Autodesk Inventor part; units mm, degrees
ref_plane "YZ Plane" through (0, 0, 0) normal (1, 0, 0) x (0, 1, 0)
ref_plane "XZ Plane" through (0, 0, 0) normal (0, 1, 0) x (-1, 0, 0)
ref_plane "XY Plane" through (0, 0, 0) normal (0, 0, 1) x (1, 0, 0)
sketch "Sketch1" plane through (0, 0, 0) normal (0, 1, 0) x (-1, 0, 0)
  point P0 (0, 0)
sketch "Sketch2" plane through (0, 0, 0) normal (0, 1, 0) x (-1, 0, 0)
  line L0 (0, 0) -> (104.775, 0)
  line L1 (104.775, 0) -> (104.775, -249.2375)
  line L2 (104.775, -249.2375) -> (0, -249.2375)
  line L3 (0, -249.2375) -> (0, 0)
  dimension "d0" = 104.775
  dimension "d1" = 249.2375
extrude "Extrusion1" add sketch "Sketch2" along normal blind 1.5875
sketch "Sketch3" plane through (0, 1.5875, 0) normal (0, 1, 0) x (1, 0, 0)
  line L0 (-104.775, 0) -> (0, 0)
  line L1 (-104.775, 0) -> (-103.1875, 0)
  line L2 (-103.1875, 0) -> (-103.1875, 304.8)
  line L3 (-104.775, 304.8) -> (-104.775, 0)
  line L4 (-104.775, 249.2375) -> (-104.775, 0)
  line L5 (-104.775, 0) -> (79.375, 0)
  line L6 (79.375, 0) -> (79.375, 1.5875)
  line L7 (79.375, 1.5875) -> (-104.775, 1.5875)
  line L8 (-104.775, 1.5875) -> (-104.775, 0)
  line L9 (0, 249.2375) -> (-104.775, 249.2375)
  line L10 (-104.775, 249.2375) -> (79.375, 249.2375)
  line L11 (79.375, 249.2375) -> (79.375, 247.65)
  line L12 (79.375, 247.65) -> (-104.775, 247.65)
  line L13 (-104.775, 247.65) -> (-104.775, 249.2375)
  line L14 (-104.775, 304.8) -> (-103.1875, 304.8)
  line L15 (-103.1875, 304.8) -> (-103.1875, 0)
  line L16 (-103.1875, 0) -> (-104.775, 0)
  line L17 (-104.775, 0) -> (-104.775, 304.8)
  dimension "d6" = 184.15
  dimension "d7" = 1.5875
  dimension "d8" = 184.15
  dimension "d9" = 1.5875
  dimension "d10" = 1.5875
  dimension "d11" = 304.8
extrude "Extrusion2" add sketch "Sketch3" along normal blind 76.2
sketch "Sketch4" plane through (-103.1875, 1.5875, -1.5875) normal (1, 0, 0) x (0, 0, -1)
  line L0 (-1.5875, -1.5875) -> (-1.5875, 0) construction
  line L1 (-1.5875, -1.5875) -> (30.1625, -1.5875) construction
  line L2 (247.65, -1.5875) -> (-1.5875, -1.5875) construction
  line L3 (30.1625, -1.5875) -> (30.1625, 0) construction
  line L4 (0, 0) -> (246.0625, 0) construction
  line L5 (0, 76.2) -> (246.0625, 76.2)
  line L6 (30.1625, 0) -> (31.75, 0)
  line L7 (31.75, 0) -> (31.75, 76.2)
  line L8 (31.75, 76.2) -> (30.1625, 76.2)
  line L9 (30.1625, 76.2) -> (30.1625, 0)
  dimension "d14" = 31.75
  dimension "d15" = 1.5875
extrude "Extrusion3" add sketch "Sketch4" along normal blind 182.5625
sketch "Sketch5" plane through (-104.775, 0, -249.2375) normal (-1, 0, 0) x (0, 0, 1)
  line L0 (-55.5625, 1.5875) -> (-55.5625, 77.7875)
  line L1 (0, 0) -> (0, 1.5875)
  line L2 (-55.5625, 77.7875) -> (0, 77.7875)
  line L3 (0, 77.7875) -> (0, 1.5875)
  line L4 (0, 1.5875) -> (-55.5625, 1.5875)
  line L5 (-55.5625, 1.5875) -> (-55.5625, 77.7875)
  point P0 (249.2375, 0)
extrude "Extrusion4" cut sketch "Sketch5" against normal blind 50.8
sketch "Sketch6" plane through (-104.775, 0, 0) normal (0, 0, 1) x (1, 0, 0)
  line L0 (184.15, 1.5875) -> (104.775, 1.5875) construction
  line L1 (106.3548, 1.5875) -> (106.3548, 49.2125) construction
  line L2 (106.3548, 1.5875) -> (153.9798, 1.5875) construction
  line L3 (184.15, 56.388) -> (92.075, 56.388) construction
  line L4 (92.075, 56.388) -> (92.075, 40.3233) construction
  circle A0 centre (92.075, 49.2125) radius 1.905 construction
  point P0 (104.775, 0)
  dimension "d20" = 47.625
  dimension "d21" = 90
  dimension "d22" = 92.075
  dimension "d23" = 3.81
properties part number "Collector Base"
The listing builds one solid part. Answer for the finished solid, in the listing's coordinates (mm). A direction names the side the tool comes from. Give positions to 0.01 mm unless a question says otherwise; leave off trailing zeros. Loops run counter-clockwise (first coordinate to the right, second up) from the corner with the lowest first, then second, coordinate; pieces in that order, holes last. Notation, with made-up numbers: M 83.5,-39.5 L 91.5,-39.5 A30 ccw 91.5,-6.5 Z; hole C 22,71.25 d1. An arc over 180 degrees is marked long. Answer as CSV lines item,"result".
Item 1: Straight lines are drawn through the part: line 1 along Z through (x, y) = (20.5, 71); line 2 along X through (y, z) = (65, -220) (1 decimal); line 3 along Y through (x, z) = (-84.5, -92.5). For each, find the intervals that lie inside material, in ascending order. Write a range as [from, to].
Values follow:
line 1,"z = [-249.24, -247.65], [-33.34, -31.75], [-1.59, 0]"
line 2,"x = [-104.8, -103.2]"
line 3,"y = [0, 1.59]"
Item 2: The part is cut by section D-D (x = -47). Give the vertices of the cut face in (y, z).
Values follow:
outline,"M 0,-249.24 L 77.79,-249.24 L 77.79,-247.65 L 1.59,-247.65 L 1.59,-33.34 L 77.79,-33.34 L 77.79,-31.75 L 1.59,-31.75 L 1.59,-1.59 L 77.79,-1.59 L 77.79,0 L 0,0 Z"
Item 3: Given pin 1 Ø6 at (y, z) = (59.5, -159) entering from +X; pin 2 Ø1 at (x, z) = (-6, -215) entering from +Y; pin 3 Ø0.5 at (x, z) = (20.5, -1) entering from -Y, each flat-ended and moving along its own axis, determine where each tip first touches the part or whether it passes through.
Values follow:
pin 1,"stops at x = -103.19"
pin 2,"stops at y = 1.59"
pin 3,"stops at y = 1.59"
Item 4: Which of the six approach directions +Z, -Z, +X, -X, +Y, -Y give full straight-line access (tool end or side, diameter ignored) to faces 4 (the flat face through (-103.188, 39, -139)), 5 (the flat face through (-52, 0, -123))?
Values follow:
face 4,"+X, +Y"
face 5,"+Z, -Z, +X, -X, -Y"
Item 5: The mould has two halves that part along Z. Classify faces 1 (the flat face through (-104.775, 38, -123)), 2 (the flat face through (-11, 38, 0)), 3 (the flat face through (-13, 40, -31.75)): released by +Z, released by -Z, zero draft, split by the parting line, or undercut.
Values follow:
face 1,"zero draft"
face 2,"released by +Z"
face 3,"undercut"
Item 6: The part is cut by section B-B (z = -134.5). Give the vertices of the cut face in (x, y) (1 decimal).
Values follow:
outline,"M -104.8,0 L 0,0 L 0,1.6 L -103.2,1.6 L -103.2,77.8 L -104.8,77.8 Z"
Item 7: The part is cut by section A-A (x = 40). Give the vertices of the cut face in (y, z), and give its area (3 significant figures).
Values follow:
outline,"M 1.59,-249.24 L 77.79,-249.24 L 77.79,-247.65 L 1.59,-247.65 Z; M 1.59,-33.34 L 77.79,-33.34 L 77.79,-31.75 L 1.59,-31.75 Z; M 1.59,-1.59 L 77.79,-1.59 L 77.79,0 L 1.59,0 Z"
area,"363 mm^2"
